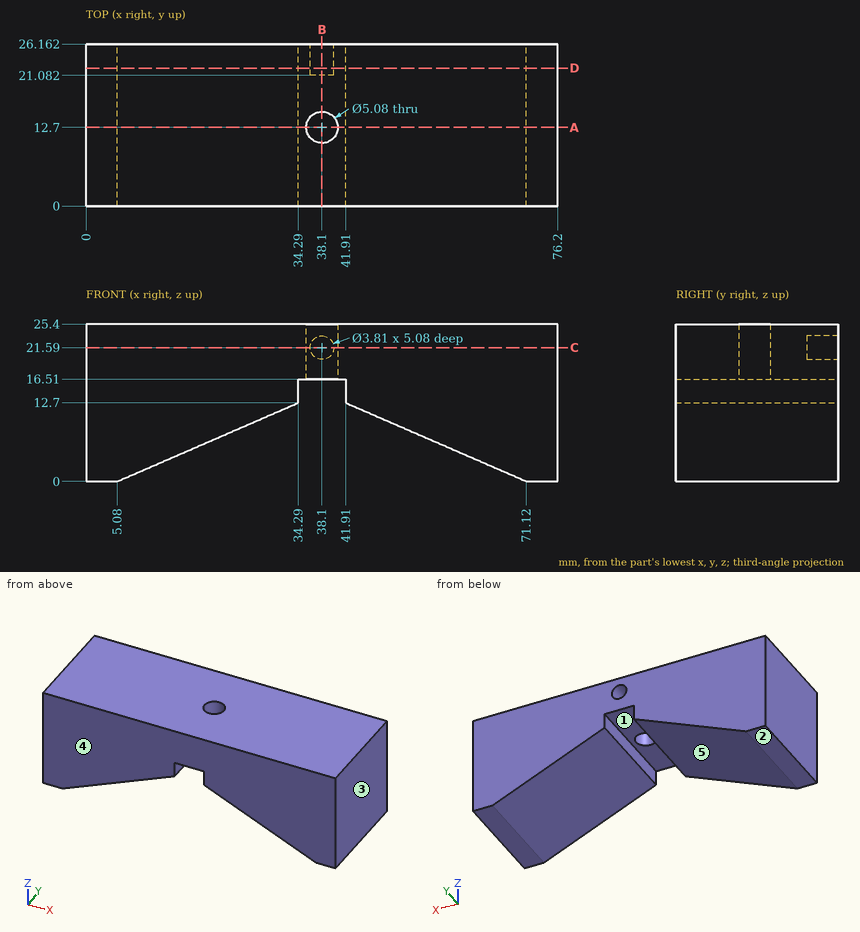
Geometry: see drawing. Coordinates: mm, zero at the bounding-box minimum. A direction names the side the tool comes from. Give positions to 0.01 mm unless a question says otherwise; leave off trailing zeros. Loops run counter-clockwise (first coordinate to the right, second up) from the corner with the lowest first, then second, coordinate; pieces in that order, holes last. Notation, with made-up numbers: M -22.75,10 L -17.75,10 A19 cw -17.75,29 Z; hole C -7,37.5 d7. An arc over 180 degrees is marked long. Answer as CSV lines item,"result". Start each with the question number.
1. Section D-D on y = 22.25. Return loops of the section in (x, z) (3 decimals).
2. Pull-direction query (X, two-part tool) for the marked faces 3, 4 and 5; classes: released by +X, released by -X, zero draft, split by the parting line, or undercut.
3. Pin query (flat end, axial travel): P1, Ø6, axis at x = 37, y = 9.5, coming from the -Z side; P2, Ø8, axis at x = 14.5, y = 15.5, coming from the -Z side. Return the tip coordinate at first contact, or that it passes through.
4. Line query: L1, parallel to Y at x = 38.1, z = 22.25; L2, parallel to X at y = 23.45, z = 21.59 (3 decimals); L3, parallel to X at y = 23.5, z = 13.5. Output: solid intervals per line, ascending.
5. Reachability of the marked faces 1 and 2 from +Z, -Z, +X, -X, +Y, -Y: full face, straight path, thin tool, end or side. Return the list, or none.
6. Section A-A on y = 12.7. Return loops of the section in (x, z).
7. Section C-C on z = 21.59. Return loops of the section in (x, y) (3 decimals), plus the area to 3 significant figures.
8. Section B-B on x = 38.1. Return loops of the section in (y, z) (3 decimals).
Computed values:
1,outline,"M 0,0 L 5.08,0 L 34.29,12.7 L 34.29,16.51 L 41.91,16.51 L 41.91,12.7 L 71.12,0 L 76.2,0 L 76.2,25.4 L 0,25.4 Z; hole C 38.1,21.59 d3.81"
2,face 3,"released by +X"
2,face 4,"zero draft"
2,face 5,"undercut"
3,P1,"stops at z = 12.57"
3,P2,"stops at z = 2.36"
4,L1,"y = 0 to 10.16, 15.24 to 21.08"
4,L2,"x = 0 to 36.195, 40.005 to 76.2"
4,L3,"x = 0 to 34.29, 41.91 to 76.2"
5,face 1,"-Z, +Y, -Y"
5,face 2,"-Z, +X, -X, +Y, -Y"
6,outline,"M 0,0 L 5.08,0 L 34.29,12.7 L 34.29,16.51 L 35.56,16.51 L 35.56,25.4 L 0,25.4 Z; M 40.64,16.51 L 41.91,16.51 L 41.91,12.7 L 71.12,0 L 76.2,0 L 76.2,25.4 L 40.64,25.4 Z"
7,outline,"M 0,0 L 76.2,0 L 76.2,26.162 L 40.005,26.162 L 40.005,21.082 L 36.195,21.082 L 36.195,26.162 L 0,26.162 Z; hole C 38.1,12.7 d5.08"
7,area,"1,950 mm²"
8,outline,"M 0,16.51 L 10.16,16.51 L 10.16,25.4 L 0,25.4 Z; M 15.24,16.51 L 26.162,16.51 L 26.162,19.685 L 21.082,19.685 L 21.082,23.495 L 26.162,23.495 L 26.162,25.4 L 15.24,25.4 Z"
